The listing builds one solid part. Answer for the finished solid, in the listing's coordinates (mm). A direction names the side the tool comes from. Give positions to 0.01 mm unless a question says otherwise; leave off trailing zeros. Write each loop counter-clockwise with the first axis right and the second up, starting at its lowest first coordinate (ties: lowest second). Pieces come first, ordered by that corner, then holes. Notation, with made-up numbers: (87.25, 86) - (100.25, 86) arc R27 ccw to (100.25, 102) - close; hole circle Ø8 at (-15.75, 44.5). An arc over 180 degrees is marked (long way). One line per question, with ' | ' between items. Start each with the question number.
1. A cutting plane is placed at D-D (x = 43.5). Determine the outline of the cut face in (y, z), then the cut area to 3 significant figures.
2. For faces 4 (the face through (2, 2, -34.5)), 5 (the face through (-47, 0, -58.5)), 6 (the face through (-31.5, 2, 0)), 7 (the face through (12, 4, -27)), 8 (the face through (-48, 2.2, 51)), determine the directions among +Z, -Z, +X, -X, +Y, -Y from which every point of the face is accessible in a straight line to the end or side of a thin tool.
3. A cutting plane is placed at B-B (x = -48.5). Determine the outline of the cut face in (y, z).
4. Given P1, Ø13.5, axis at x = -51, z = -51, coming from the -Y side; P2, Ø4.5, axis at x = 55, y = 2, coming from the +Z side; P3, Ø1, axis at x = 18, y = 1.5, coming from the +Z side; P4, Ø10, axis at x = -48.5, z = -50.5, coming from the -Y side, each flat-ended and moving along its own axis, determine where each tip first touches the part or whether it passes through.
5. The mould has two halves that part along X. Classify faces 1 (the face through (-41.5, 2, 1)), 2 (the face through (43, 0, 58.5)), 3 (the face through (-30.5, 2, 47)): +X half, -X half, draft (parallel to the pull), parting line (faces both ways), or undercut.
6. Find the intervals of material crossed by L1, parallel to X at y = 0.25, z = 50.5; L2, parallel to X at y = -2.5, z = 49.5; L3, parallel to Z at x = 32.5, y = 1, in increasing order. Write a range as from..to.
7. A cutting plane is placed at A-A (y = -2.25). State how many separate pieces and enclosed holes the cut face has, then the cut area to 3 significant figures.
```python
from build123d import *

# Parameters (mm, degrees)
SKETCH1_W                       = 113
SKETCH1_H                       = 85
BOSS_EXTRUDE1_DEPTH             = 4
SKETCH2_R                       = 1.5
CUT_EXTRUDE1_DEPTH              = 71.813134375
BOSS_EXTRUDE3_REACH             = 72.813
SKETCH4_W                       = 16
SKETCH4_H                       = 16
BOSS_EXTRUDE3_DIRECTION_2_DEPTH = 1
SKETCH10_W                      = 10
SKETCH10_H                      = 16
BOSS_EXTRUDE6_DEPTH             = 4
SKETCH6_W                       = 73
SKETCH6_H                       = 45
SKETCH6_W_2                     = 15
SKETCH6_H_2                     = 85
SKETCH6_W_3                     = 66
SKETCH6_H_3                     = 8
CUT_EXTRUDE2_DEPTH              = 82.483127088
SKETCH8_R                       = 6.1
CUT_EXTRUDE3_DEPTH              = 3.2
SKETCH9_W                       = 16
SKETCH9_H                       = 16
SKETCH9_W_2                     = 14
SKETCH9_H_2                     = 14
BOSS_EXTRUDE5_DEPTH             = 3
FILLET1_R                       = 0.2


with BuildPart() as part:
    # Sketch1 → Boss-Extrude1 (new body)
    with BuildSketch(Plane(origin=(0, 0, 0), x_dir=(1, 0, 0), z_dir=(0, 1, 0))):
        Rectangle(SKETCH1_W, SKETCH1_H)
    extrude(amount=BOSS_EXTRUDE1_DEPTH)

    # Sketch2 → Cut-Extrude1 (cut, through all)
    with BuildSketch(Plane(origin=(0, 4, 0), x_dir=(1, 0, 0), z_dir=(0, 1, 0))):
        with Locations(Location((-18.75, 28, 0), (0, 0, 270))):
            Circle(SKETCH2_R)
        with Locations(Location((-18.75, -28, 0), (0, 0, 270))):
            Circle(SKETCH2_R)
        with Locations(Location((51.25, -20, 0), (0, 0, 270))):
            Circle(SKETCH2_R)
        with Locations(Location((51.25, 20, 0), (0, 0, 270))):
            Circle(SKETCH2_R)
    extrude(amount=-CUT_EXTRUDE1_DEPTH, mode=Mode.SUBTRACT)

    # Boss-Extrude3: up to this face of the body (flat: up to its plane)
    boss_extrude3_end = Plane(part.part.faces().sort_by_distance((-0.047976515, 4, 0))[0])
    # Sketch4 → Boss-Extrude3 (add, up to the picked face)
    with BuildSketch(Plane.XZ, mode=Mode.PRIVATE) as boss_extrude3_sk1:
        with Locations((-48.5, 50.5)):
            Rectangle(SKETCH4_W, SKETCH4_H)
    boss_extrude3_tool1 = split(extrude(boss_extrude3_sk1.sketch, amount=-BOSS_EXTRUDE3_REACH, mode=Mode.PRIVATE), bisect_by=boss_extrude3_end, keep=Keep.BOTH, mode=Mode.PRIVATE)
    # Sketch4 → Boss-Extrude3 (add, up to the picked face)
    with BuildSketch(Plane.XZ, mode=Mode.PRIVATE) as boss_extrude3_sk2:
        with Locations((43.5, 50.5)):
            Rectangle(SKETCH4_W, SKETCH4_H)
    boss_extrude3_tool2 = split(extrude(boss_extrude3_sk2.sketch, amount=-BOSS_EXTRUDE3_REACH, mode=Mode.PRIVATE), bisect_by=boss_extrude3_end, keep=Keep.BOTH, mode=Mode.PRIVATE)
    # Sketch4 → Boss-Extrude3 (add, up to the picked face)
    with BuildSketch(Plane.XZ, mode=Mode.PRIVATE) as boss_extrude3_sk3:
        with Locations((43.5, -50.5)):
            Rectangle(SKETCH4_W, SKETCH4_H)
    boss_extrude3_tool3 = split(extrude(boss_extrude3_sk3.sketch, amount=-BOSS_EXTRUDE3_REACH, mode=Mode.PRIVATE), bisect_by=boss_extrude3_end, keep=Keep.BOTH, mode=Mode.PRIVATE)
    # Sketch4 → Boss-Extrude3 (add, up to the picked face)
    with BuildSketch(Plane.XZ, mode=Mode.PRIVATE) as boss_extrude3_sk4:
        with Locations((-48.5, -50.5)):
            Rectangle(SKETCH4_W, SKETCH4_H)
    boss_extrude3_tool4 = split(extrude(boss_extrude3_sk4.sketch, amount=-BOSS_EXTRUDE3_REACH, mode=Mode.PRIVATE), bisect_by=boss_extrude3_end, keep=Keep.BOTH, mode=Mode.PRIVATE)
    add(boss_extrude3_tool1.solids().sort_by(Axis((-48.5, 0, 50.5), (0, 1, 0)))[0])
    add(boss_extrude3_tool2.solids().sort_by(Axis((43.5, 0, 50.5), (0, 1, 0)))[0])
    add(boss_extrude3_tool3.solids().sort_by(Axis((43.5, 0, -50.5), (0, 1, 0)))[0])
    add(boss_extrude3_tool4.solids().sort_by(Axis((-48.5, 0, -50.5), (0, 1, 0)))[0])

    # Sketch4 → Boss-Extrude3 direction 2 (add)
    with BuildSketch(Plane.XZ):
        with Locations((-48.5, 50.5)):
            Rectangle(SKETCH4_W, SKETCH4_H)
        with Locations((43.5, 50.5)):
            Rectangle(SKETCH4_W, SKETCH4_H)
        with Locations((43.5, -50.5)):
            Rectangle(SKETCH4_W, SKETCH4_H)
        with Locations((-48.5, -50.5)):
            Rectangle(SKETCH4_W, SKETCH4_H)
    extrude(amount=BOSS_EXTRUDE3_DIRECTION_2_DEPTH)

    # Sketch10 → Boss-Extrude6 (add)
    with BuildSketch(Plane(origin=(0, 4, 0), x_dir=(1, 0, 0), z_dir=(0, 1, 0))):
        with Locations((-35.5, -50.5)):
            Rectangle(SKETCH10_W, SKETCH10_H)
        with Locations((-35.5, 50.5)):
            Rectangle(SKETCH10_W, SKETCH10_H)
    extrude(amount=-BOSS_EXTRUDE6_DEPTH)

    # Sketch6 → Cut-Extrude2 (cut, through all)
    with BuildSketch(Plane(origin=(0, 4, 0), x_dir=(1, 0, 0), z_dir=(0, 1, 0))):
        with Locations((5, 0)):
            Rectangle(SKETCH6_W, SKETCH6_H)
        with Locations((-49, 0)):
            Rectangle(SKETCH6_W_2, SKETCH6_H_2)
        with Locations((2.5, 38.5)):
            Rectangle(SKETCH6_W_3, SKETCH6_H_3)
        with Locations((2.5, -38.5)):
            Rectangle(SKETCH6_W_3, SKETCH6_H_3)
    extrude(amount=-CUT_EXTRUDE2_DEPTH, mode=Mode.SUBTRACT)

    # Sketch8 → Cut-Extrude3 (cut)
    with BuildSketch(Plane.XZ.offset(1)):
        with Locations(Location((-48.5, 50.5, 0), (0, 0, 270))):
            Circle(SKETCH8_R)
        with Locations(Location((43.5, 50.5, 0), (0, 0, 270))):
            Circle(SKETCH8_R)
        with Locations(Location((43.5, -50.5, 0), (0, 0, 90))):
            Circle(SKETCH8_R)
        with Locations(Location((-48.5, -50.5, 0), (0, 0, 90))):
            Circle(SKETCH8_R)
    extrude(amount=-CUT_EXTRUDE3_DEPTH, mode=Mode.SUBTRACT)

    # Sketch9 → Boss-Extrude5 (add)
    # profile 1 of 4: a face of its own
    with BuildSketch(Plane.XZ.offset(1)):
        with Locations((-48.5, 50.5)):
            Rectangle(SKETCH9_W, SKETCH9_H)
        with Locations((-48.5, 50.5)):
            Rectangle(SKETCH9_W_2, SKETCH9_H_2, mode=Mode.SUBTRACT)
    # profile 2 of 4: a face of its own
    with BuildSketch(Plane.XZ.offset(1)):
        with Locations((43.5, 50.5)):
            Rectangle(SKETCH9_W, SKETCH9_H)
        with Locations((43.5, 50.5)):
            Rectangle(SKETCH9_W_2, SKETCH9_H_2, mode=Mode.SUBTRACT)
    # profile 3 of 4: a face of its own
    with BuildSketch(Plane.XZ.offset(1)):
        with Locations((43.5, -50.5)):
            Rectangle(SKETCH9_W, SKETCH9_H)
        with Locations((43.5, -50.5)):
            Rectangle(SKETCH9_W_2, SKETCH9_H_2, mode=Mode.SUBTRACT)
    # profile 4 of 4: a face of its own
    with BuildSketch(Plane.XZ.offset(1)):
        with Locations((-48.5, -50.5)):
            Rectangle(SKETCH9_W, SKETCH9_H)
        with Locations((-48.5, -50.5)):
            Rectangle(SKETCH9_W_2, SKETCH9_H_2, mode=Mode.SUBTRACT)
    extrude(amount=BOSS_EXTRUDE5_DEPTH)

    # Fillet1
    fillet1_edges = [part.edges().sort_by_distance(p)[0] for p in [
        (-48.5, -1, -56.6),
        (43.5, -1, -56.6),
        (43.5, -1, 56.6),
        (-48.5, -1, 56.6),
    ]]
    fillet(fillet1_edges, radius=FILLET1_R)


solid = part.part
```
Determined:
1) outline: (-4, -58.5) - (4, -58.5) - (4, 58.5) - (-4, 58.5) - (-4, 57.5) - (-1, 57.5) - (-1, 56.8) arc R0.2 ccw to (-0.8, 56.6) - (2.2, 56.6) - (2.2, 44.4) - (-0.8, 44.4) arc R0.2 ccw to (-1, 44.2) - (-1, 43.5) - (-4, 43.5) - (-4, 42.5) - (0, 42.5) - (0, -42.5) - (-4, -42.5) - (-4, -43.5) - (-1, -43.5) - (-1, -44.2) arc R0.2 ccw to (-0.8, -44.4) - (2.2, -44.4) - (2.2, -56.6) - (-0.8, -56.6) arc R0.2 ccw to (-1, -56.8) - (-1, -57.5) - (-4, -57.5) - close | area: 434 mm2
2) face 4: -Z, +Y, -Y | face 5: -Z, +X, -X, +Y, -Y | face 6: +Y, -Y | face 7: +Z, -Z, +X, -X, +Y | face 8: -Y
3) outline: (-4, -58.5) - (4, -58.5) - (4, -42.5) - (-4, -42.5) - (-4, -43.5) - (-1, -43.5) - (-1, -44.2) arc R0.2 ccw to (-0.8, -44.4) - (2.2, -44.4) - (2.2, -56.6) - (-0.8, -56.6) arc R0.2 ccw to (-1, -56.8) - (-1, -57.5) - (-4, -57.5) - close; (-4, 42.5) - (4, 42.5) - (4, 58.5) - (-4, 58.5) - (-4, 57.5) - (-1, 57.5) - (-1, 56.8) arc R0.2 ccw to (-0.8, 56.6) - (2.2, 56.6) - (2.2, 44.4) - (-0.8, 44.4) arc R0.2 ccw to (-1, 44.2) - (-1, 43.5) - (-4, 43.5) - close
4) P1: y = -4 | P2: z = 42.5 | P3: z = 34.5 | P4: y = 2.2
5) face 1: -X half | face 2: draft | face 3: undercut
6) L1: -56.5..-54.6, -42.4..-30.5, 35.5..37.4, 49.6..51.5 | L2: -56.5..-55.5, -41.5..-40.5, 35.5..36.5, 50.5..51.5 | L3: -34.5..-22.5, 22.5..34.5
7) separate pieces: 4 | enclosed holes: 4 | area: 240 mm2
